from build123d import *

# Parameters (mm, degrees)
RESSALTO_EXTRUS_O1_DEPTH = 31.8
RESSALTO_EXTRUS_O2_START = 31.8
RESSALTO_EXTRUS_O2_DEPTH = 168.2
FILETE1_R                = 80
FILETE2_R                = 30
FILETE3_R                = 70
ESBO_O2_R                = 1.6
CORTE_EXTRUS_O2_DEPTH    = 228.870577403


with BuildPart() as part:
    # Esboço1 → Ressalto-extrusão1 (new body)
    with BuildSketch(Plane.XY):
        Polygon((-17.8, 75), (-25, 75), (-25, 105), (-30, 105), (-30, 75), (-30, 0), (-12.8, 0), (-12.8, 75), (-12.8, 105), (-17.8, 105), align=None)
        with BuildLine():
            Line((-12.8, 0), (-30, 0))
            Line((-30, 0), (-30, -42.598518169))
            ThreePointArc((-30, -42.598518169), (-3.119977625, -64.576731192), (30, -75))
            ThreePointArc((30, -75), (-2.613275136, -43.899042345), (-12.8, 0))
        make_face()
    extrude(amount=RESSALTO_EXTRUS_O1_DEPTH)

    # Esboço1<4> → Ressalto-extrusão2 (add)
    with BuildSketch(Plane.XY.offset(RESSALTO_EXTRUS_O2_START)):
        with BuildLine():
            Line((-12.8, 0), (-30, 0))
            Line((-30, 0), (-30, -42.598518169))
            ThreePointArc((-30, -42.598518169), (-3.119977625, -64.576731192), (30, -75))
            ThreePointArc((30, -75), (-2.613275136, -43.899042345), (-12.8, 0))
        make_face()
    extrude(amount=RESSALTO_EXTRUS_O2_DEPTH)

    # Filete1
    # the kernel refuses this fillet: 80 mm, written as the material it adds along each edge
    with BuildSketch(Plane(origin=(-12.8, 0, 31.8), x_dir=(0, 0, 1), z_dir=(-1, 0, 0))) as filete1_piece_1_section:
        with BuildLine():
            CenterArc((FILETE1_R, FILETE1_R), FILETE1_R, 180, 90)
            Line((0, FILETE1_R), (0, 0))
            Line((0, 0), (FILETE1_R, 0))
        make_face()
    filete1_piece_1 = extrude(amount=17.2, mode=Mode.PRIVATE)
    filete1_piece_1 = filete1_piece_1 - Plane(origin=(65.698057665, -4.916041759, 49.992599302), x_dir=(-0.4538743908259289, -0.8910656751061574, 0), z_dir=(0, 0, -1)) * Cylinder(78.65184374, 355, mode=Mode.PRIVATE)
    filete1_piece_1 = split(filete1_piece_1, bisect_by=Plane(origin=(-15.301775564, 75, 49.992599302), z_dir=(0, -1, 0)), keep=Keep.TOP, mode=Mode.PRIVATE)
    filete1_piece_1 = split(filete1_piece_1, bisect_by=Plane(origin=(-17.8, 17.823232591, 49.992599302), z_dir=(1, 0, 0)), keep=Keep.TOP, mode=Mode.PRIVATE)
    add(filete1_piece_1)
    with BuildSketch(Plane(origin=(-12.8, 0, 31.8), x_dir=(0, 0, 1), z_dir=(-1, 0, 0))) as filete1_piece_2_section:
        with BuildLine():
            CenterArc((FILETE1_R, FILETE1_R), FILETE1_R, 180, 90)
            Line((0, FILETE1_R), (0, 0))
            Line((0, 0), (FILETE1_R, 0))
        make_face()
    filete1_piece_2 = extrude(amount=17.2, mode=Mode.PRIVATE)
    filete1_piece_2 = split(filete1_piece_2, bisect_by=Plane(origin=(-15.3, 75, 31.026714825), z_dir=(0, 1, 0)), keep=Keep.TOP, mode=Mode.PRIVATE)
    filete1_piece_2 = split(filete1_piece_2, bisect_by=Plane(origin=(-17.8, 77.46056258, 31.026714825), z_dir=(1, 0, 0)), keep=Keep.TOP, mode=Mode.PRIVATE)
    add(filete1_piece_2)
    with BuildSketch(Plane(origin=(-12.8, 0, 31.8), x_dir=(0, 0, 1), z_dir=(-1, 0, 0))) as filete1_piece_3_section:
        with BuildLine():
            CenterArc((FILETE1_R, FILETE1_R), FILETE1_R, 180, 90)
            Line((0, FILETE1_R), (0, 0))
            Line((0, 0), (FILETE1_R, 0))
        make_face()
    filete1_piece_3 = extrude(amount=17.2, mode=Mode.PRIVATE)
    filete1_piece_3 = split(filete1_piece_3, bisect_by=Plane(origin=(-25, 17.809681015, 50.007682963), z_dir=(1, 0, 0)), keep=Keep.TOP, mode=Mode.PRIVATE)
    filete1_piece_3 = split(filete1_piece_3, bisect_by=Plane(origin=(-21.4, 75, 50.007682963), z_dir=(0, -1, 0)), keep=Keep.TOP, mode=Mode.PRIVATE)
    filete1_piece_3 = split(filete1_piece_3, bisect_by=Plane(origin=(-17.8, 17.809681015, 50.007682963), z_dir=(-1, 0, 0)), keep=Keep.TOP, mode=Mode.PRIVATE)
    add(filete1_piece_3)
    with BuildSketch(Plane(origin=(-12.8, 0, 31.8), x_dir=(0, 0, 1), z_dir=(-1, 0, 0))) as filete1_piece_4_section:
        with BuildLine():
            CenterArc((FILETE1_R, FILETE1_R), FILETE1_R, 180, 90)
            Line((0, FILETE1_R), (0, 0))
            Line((0, 0), (FILETE1_R, 0))
        make_face()
    filete1_piece_4 = extrude(amount=17.2, mode=Mode.PRIVATE)
    filete1_piece_4 = split(filete1_piece_4, bisect_by=Plane(origin=(-25, 17.809681015, 50.007682963), z_dir=(-1, 0, 0)), keep=Keep.TOP, mode=Mode.PRIVATE)
    filete1_piece_4 = split(filete1_piece_4, bisect_by=Plane(origin=(-27.5, 75, 50.007682963), z_dir=(0, -1, 0)), keep=Keep.TOP, mode=Mode.PRIVATE)
    add(filete1_piece_4)
    with BuildSketch(Plane(origin=(-12.8, 0, 31.8), x_dir=(0, 0, 1), z_dir=(-1, 0, 0))) as filete1_piece_5_section:
        with BuildLine():
            CenterArc((FILETE1_R, FILETE1_R), FILETE1_R, 180, 90)
            Line((0, FILETE1_R), (0, 0))
            Line((0, 0), (FILETE1_R, 0))
        make_face()
    filete1_piece_5 = extrude(amount=17.2, mode=Mode.PRIVATE)
    filete1_piece_5 = split(filete1_piece_5, bisect_by=Plane(origin=(-25, 77.46056258, 31.026714825), z_dir=(-1, 0, 0)), keep=Keep.TOP, mode=Mode.PRIVATE)
    filete1_piece_5 = split(filete1_piece_5, bisect_by=Plane(origin=(-27.5, 75, 31.026714825), z_dir=(0, 1, 0)), keep=Keep.TOP, mode=Mode.PRIVATE)
    add(filete1_piece_5)

    # Filete2
    filete2_edges = [part.edges().sort_by_distance(p)[0] for p in [
        (-30, -42.598518169, 100),
    ]]
    fillet(filete2_edges, radius=FILETE2_R)

    # Filete3
    # the kernel refuses this fillet: 70 mm, written as the material it takes off along each edge
    with BuildSketch(Plane(origin=(162.2, 0, 200), x_dir=(0, -1, 0), z_dir=(-1, 0, 0))) as filete3_piece_1:
        with BuildLine():
            CenterArc((FILETE3_R, -FILETE3_R), FILETE3_R, 90, 90)
            Line((0, -FILETE3_R), (0, 0))
            Line((0, 0), (FILETE3_R, 0))
        make_face()
    extrude(amount=367.2, mode=Mode.SUBTRACT)

    # Esboço2 → Corte-extrusão2 (cut, through all)
    with BuildSketch(Plane(origin=(0, 0, 0), x_dir=(0, 0, -1), z_dir=(1, 0, 0))):
        with Locations((-23.85, 90)):
            Circle(ESBO_O2_R)
        with Locations((-7.95, 90)):
            Circle(ESBO_O2_R)
        Polygon((-187.539156299, -70), (-160.893258266, -56.677050983), (-160.893258266, -70), align=None)
        Polygon((-190.893258266, -68.322949017), (-164.247360232, -55), (-190.893258266, -55), align=None)
    extrude(amount=-CORTE_EXTRUS_O2_DEPTH, mode=Mode.SUBTRACT)


solid = part.part
Can you work these out from the model? Positions are in its coordinate system, mm. A direction names the side the tool comes from. Round coordinates to 2 decimals unless told otherwise and drop trailing zeros. Write each loop counter-clockwise with the first axis right and the second up, starting at its lowest first coordinate (ties: lowest second). Pieces come first, ordered by that corner, then holes. Notation, with made-up numbers: M 47,75.25 L 54,75.25 A13 cw 54,98.25 Z; hole C 44,88.25 d10. An arc over 180 degrees is marked long. Use a Markdown table: item, result.
Item 1: I want a section at B-B (x = -5.5). List the corners of the cut face in (y, z) for me.
Found:
| item | result |
|---|---|
| outline | M -63.25,0 L -38.34,0 L -38.34,192.43 A70 ccw -63.25,199.67 L -63.25,190.89 L -55,190.89 L -55,164.25 L -63.25,180.74 L -63.25,174.03 L -56.68,160.89 L -63.25,160.89 Z |
Item 2: I want a section at C-C (y = -11.5). List the corners of the cut face in (x, z) for me, and give its area (3 significant figures).
Found:
| item | result |
|---|---|
| outline | M -30,0 L -12.68,0 L -12.68,168.44 L -30,168.44 Z |
| area | 2,920 mm2 |
Item 3: I want a section at A-A (z = 18). List the corners of the cut face in (x, y) for me.
Found:
| item | result |
|---|---|
| outline | M -30,-30.48 A30 ccw -19.66,-53.14 A91.8 ccw 30,-75 A78.65 cw -12.8,0 L -12.8,105 L -17.8,105 L -17.8,75 L -25,75 L -25,105 L -30,105 Z |
Item 4: We'd pull the mould along X, two halves only. Please class faces 5 (the face through (-2.294, -44.454, 98.6)), 6 (the face through (-25, 90, 16)), 7 (the face through (0, -63, 166)): released by +X, released by -X, zero draft, split by the parting line, or undercut.
Found:
| item | result |
|---|---|
| face 5 | released by +X |
| face 6 | undercut |
| face 7 | released by -X |
Item 5: Which directions (+Z, -Z, +X, -X, +Y, -Y) give clear straight access to the entire face, cutting with the end or side of a thin tool? Please do faces 1 (the face through (-7, -59, 190.893)), 2 (the face through (0, -59, 181)), 3 (the face through (-17.8, 90, 16)), 4 (the face through (-28, 93, 31.8)).
Found:
| item | result |
|---|---|
| face 1 | -X, -Y |
| face 2 | -X |
| face 3 | +Z, -Z, +Y |
| face 4 | +Z, +X, -X, +Y |
Item 6: For pin 1 Ø5.5 at (x, y) = (-15.5, 92.5) entering from +Z; pin 2 Ø12 at (x, z) = (8.5, 92.5) entering from +Y; pin 3 Ø19 at (x, z) = (-18.5, 125) entering from +Y, each with a flat end and sliding along its axis, tell me the tip position at first contact or that it passes through.
Found:
| item | result |
|---|---|
| pin 1 | stops at z = 31.8 |
| pin 2 | stops at y = -51.74 |
| pin 3 | stops at y = 0 |
Item 7: If I drill on line 1 along Z through (x, y) = (-14, 90); line 2 along Z through (x, y) = (-16, 93); line 3 along Y through (x, z) = (-27, 23), over which ranges is the centre line in solid material (lowest first)? Write a range as [from, to].
Found:
| item | result |
|---|---|
| line 1 | z = [0, 6.35], [9.55, 22.25], [25.45, 31.8] |
| line 2 | z = [0, 31.8] |
| line 3 | y = [-43.56, 88.64], [91.36, 105] |
Item 8: I want a section at D-D (z = 143). List the corners of the cut face in (x, y) for me.
Found:
| item | result |
|---|---|
| outline | M -30,-30.48 A30 ccw -19.66,-53.14 A91.8 ccw 30,-75 A78.65 cw -12.87,-1.22 L -30,-1.22 Z |
